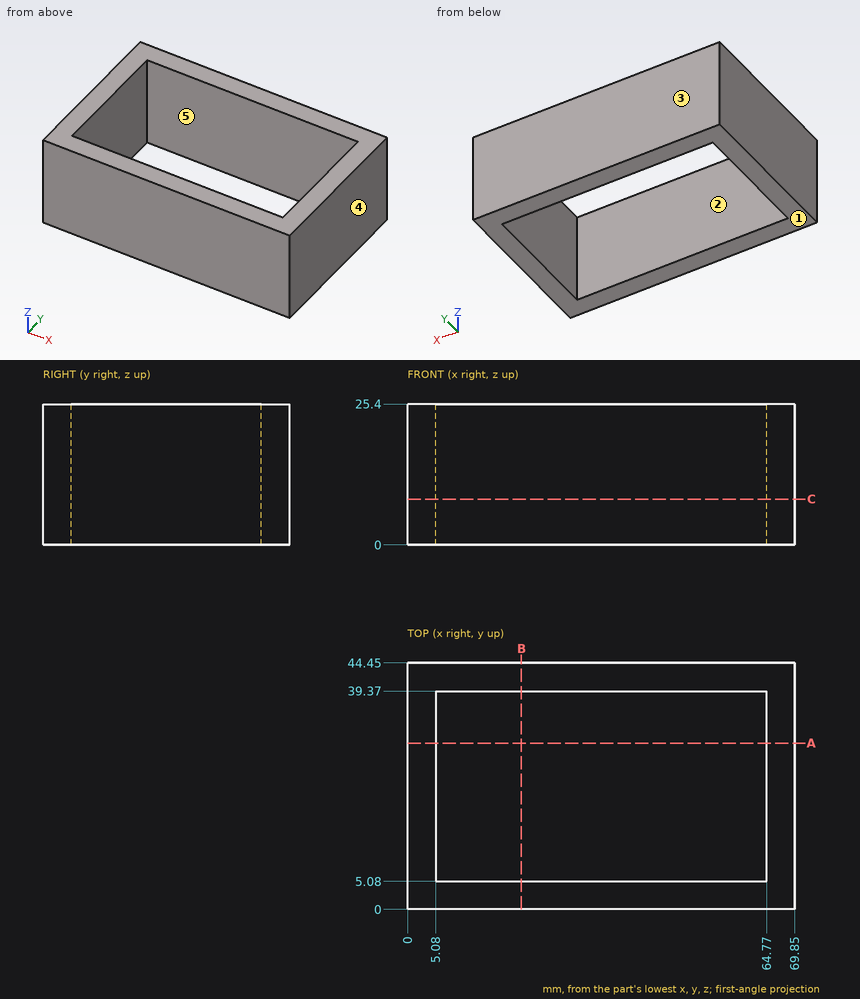
Source: three-view drawing plus pictorial views. Frame: mm from the lowest corner of the part. A direction names the side the tool comes from. Give positions to 0.01 mm unless a question says otherwise; leave off trailing zeros. Write each loop counter-clockwise with the first axis right and the second up, starting at its lowest first coordinate (ties: lowest second). Pieces come first, ordered by that corner, then holes.
(1) Ray query, line 1 (Y direction, x = 46, z = 12); line 2 (X direction, y = 7.5, z = 14). Return the intervals inside material, ascending.
(2) Access query for the marked faces 1 and 2. Directions: +Z, -Z, +X, -X, +Y, -Y. A direction counts if a zero-diameter tool reaches every point of the face in a straight line with its end or side. Return the directions, or none.
(3) Cut plane B-B, the plane x = 20.5. Return loops of the section in (y, z), then the cut area to 3 significant figures.
(4) Cut plane C-C, the plane z = 8.25. Return loops of the section in (x, y), then the cut area to 3 significant figures.
(5) Cut plane A-A, the plane y = 30. Return loops of the section in (x, z).
(6) Mould query, pull axis X, two halves, no side actions, for the marked faces 3, 4 and 5. Classes: released by +X, released by -X, zero draft, split by the parting line, or undercut.
Values follow:
1. line 1: y = 0 to 5.08, 39.37 to 44.45
1. line 2: x = 0 to 5.08, 64.77 to 69.85
2. face 1: -Z, +X, -X, +Y, -Y
2. face 2: +Z, -Z
3. outline: (0, 0) - (5.08, 0) - (5.08, 25.4) - (0, 25.4) - close; (39.37, 0) - (44.45, 0) - (44.45, 25.4) - (39.37, 25.4) - close
3. area: 258 mm2
4. outline: (0, 0) - (69.85, 0) - (69.85, 44.45) - (0, 44.45) - close; hole (5.08, 5.08) - (64.77, 5.08) - (64.77, 39.37) - (5.08, 39.37) - close
4. area: 1,060 mm2
5. outline: (0, 0) - (5.08, 0) - (5.08, 25.4) - (0, 25.4) - close; (64.77, 0) - (69.85, 0) - (69.85, 25.4) - (64.77, 25.4) - close
6. face 3: zero draft
6. face 4: released by +X
6. face 5: undercut
